```python
from build123d import *

# Parameters (mm, degrees)
ESQUISSE1_W               = 60
ESQUISSE1_H               = 70
T_LE_DE_BASE_PLI_E1_DEPTH = 3
ENL_V_MAT_EXTRU_1_REACH   = 48.195
ESQUISSE6_R               = 2
ENL_V_MAT_EXTRU_2_REACH   = 48.195
ESQUISSE7_R               = 2
BOSS_EXTRU_1_START        = 4
ESQUISSE9_R               = 4
ESQUISSE9_R_2             = 2
BOSS_EXTRU_1_DEPTH        = 4
ENL_V_MAT_EXTRU_3_REACH   = 48.271
ESQUISSE10_W              = 45
ESQUISSE10_H              = 35
BOSS_EXTRU_2_START        = -1
ESQUISSE11_R              = 2
BOSS_EXTRU_2_DEPTH        = 1
BOSS_EXTRU_3_START        = 3
ESQUISSE12_R              = 4
ESQUISSE12_R_2            = 2
BOSS_EXTRU_3_DEPTH        = 3
BOSS_EXTRU_4_START        = 1
ESQUISSE13_R              = 4
BOSS_EXTRU_4_DEPTH        = 1


# Sheet-metal steps are written as plain solids
with BuildPart() as part:
    # Esquisse1 → Tôle de base pliée1 (new body)
    with BuildSketch(Plane.XY):
        Rectangle(ESQUISSE1_W, ESQUISSE1_H)
    extrude(amount=-T_LE_DE_BASE_PLI_E1_DEPTH)

    # Esquisse6 → Enlèv. mat.-Extru.1 (cut, up to next)
    with BuildSketch(Plane.XY, mode=Mode.PRIVATE) as enl_v_mat_extru_1_sk1:
        with Locations((-24.5, 29)):
            Circle(ESQUISSE6_R)
    enl_v_mat_extru_1_tool1 = extrude(enl_v_mat_extru_1_sk1.sketch, amount=-ENL_V_MAT_EXTRU_1_REACH, mode=Mode.PRIVATE) & part.part
    # Esquisse6 → Enlèv. mat.-Extru.1 (cut, up to next)
    with BuildSketch(Plane.XY, mode=Mode.PRIVATE) as enl_v_mat_extru_1_sk2:
        with Locations((24.5, 29)):
            Circle(ESQUISSE6_R)
    enl_v_mat_extru_1_tool2 = extrude(enl_v_mat_extru_1_sk2.sketch, amount=-ENL_V_MAT_EXTRU_1_REACH, mode=Mode.PRIVATE) & part.part
    # Esquisse6 → Enlèv. mat.-Extru.1 (cut, up to next)
    with BuildSketch(Plane.XY, mode=Mode.PRIVATE) as enl_v_mat_extru_1_sk3:
        with Locations((24.5, -29)):
            Circle(ESQUISSE6_R)
    enl_v_mat_extru_1_tool3 = extrude(enl_v_mat_extru_1_sk3.sketch, amount=-ENL_V_MAT_EXTRU_1_REACH, mode=Mode.PRIVATE) & part.part
    # Esquisse6 → Enlèv. mat.-Extru.1 (cut, up to next)
    with BuildSketch(Plane.XY, mode=Mode.PRIVATE) as enl_v_mat_extru_1_sk4:
        with Locations((-24.5, -29)):
            Circle(ESQUISSE6_R)
    enl_v_mat_extru_1_tool4 = extrude(enl_v_mat_extru_1_sk4.sketch, amount=-ENL_V_MAT_EXTRU_1_REACH, mode=Mode.PRIVATE) & part.part
    add(enl_v_mat_extru_1_tool1.solids().sort_by_distance((-24.5, 29, 0))[0], mode=Mode.SUBTRACT)
    add(enl_v_mat_extru_1_tool2.solids().sort_by_distance((24.5, 29, 0))[0], mode=Mode.SUBTRACT)
    add(enl_v_mat_extru_1_tool3.solids().sort_by_distance((24.5, -29, 0))[0], mode=Mode.SUBTRACT)
    add(enl_v_mat_extru_1_tool4.solids().sort_by_distance((-24.5, -29, 0))[0], mode=Mode.SUBTRACT)

    # Esquisse7 → Enlèv. mat.-Extru.2 (cut, up to next)
    with BuildSketch(Plane.XY, mode=Mode.PRIVATE) as enl_v_mat_extru_2_sk1:
        with Locations((-17, -23.75)):
            Circle(ESQUISSE7_R)
    enl_v_mat_extru_2_tool1 = extrude(enl_v_mat_extru_2_sk1.sketch, amount=-ENL_V_MAT_EXTRU_2_REACH, mode=Mode.PRIVATE) & part.part
    # Esquisse7 → Enlèv. mat.-Extru.2 (cut, up to next)
    with BuildSketch(Plane.XY, mode=Mode.PRIVATE) as enl_v_mat_extru_2_sk2:
        with Locations((0, -23.75)):
            Circle(ESQUISSE7_R)
    enl_v_mat_extru_2_tool2 = extrude(enl_v_mat_extru_2_sk2.sketch, amount=-ENL_V_MAT_EXTRU_2_REACH, mode=Mode.PRIVATE) & part.part
    # Esquisse7 → Enlèv. mat.-Extru.2 (cut, up to next)
    with BuildSketch(Plane.XY, mode=Mode.PRIVATE) as enl_v_mat_extru_2_sk3:
        with Locations((17, -23.75)):
            Circle(ESQUISSE7_R)
    enl_v_mat_extru_2_tool3 = extrude(enl_v_mat_extru_2_sk3.sketch, amount=-ENL_V_MAT_EXTRU_2_REACH, mode=Mode.PRIVATE) & part.part
    # Esquisse7 → Enlèv. mat.-Extru.2 (cut, up to next)
    with BuildSketch(Plane.XY, mode=Mode.PRIVATE) as enl_v_mat_extru_2_sk4:
        with Locations((0, 23.75)):
            Circle(ESQUISSE7_R)
    enl_v_mat_extru_2_tool4 = extrude(enl_v_mat_extru_2_sk4.sketch, amount=-ENL_V_MAT_EXTRU_2_REACH, mode=Mode.PRIVATE) & part.part
    # Esquisse7 → Enlèv. mat.-Extru.2 (cut, up to next)
    with BuildSketch(Plane.XY, mode=Mode.PRIVATE) as enl_v_mat_extru_2_sk5:
        with Locations((17, 23.75)):
            Circle(ESQUISSE7_R)
    enl_v_mat_extru_2_tool5 = extrude(enl_v_mat_extru_2_sk5.sketch, amount=-ENL_V_MAT_EXTRU_2_REACH, mode=Mode.PRIVATE) & part.part
    # Esquisse7 → Enlèv. mat.-Extru.2 (cut, up to next)
    with BuildSketch(Plane.XY, mode=Mode.PRIVATE) as enl_v_mat_extru_2_sk6:
        with Locations((-17, 23.75)):
            Circle(ESQUISSE7_R)
    enl_v_mat_extru_2_tool6 = extrude(enl_v_mat_extru_2_sk6.sketch, amount=-ENL_V_MAT_EXTRU_2_REACH, mode=Mode.PRIVATE) & part.part
    add(enl_v_mat_extru_2_tool1.solids().sort_by_distance((-17, -23.75, 0))[0], mode=Mode.SUBTRACT)
    add(enl_v_mat_extru_2_tool2.solids().sort_by_distance((0, -23.75, 0))[0], mode=Mode.SUBTRACT)
    add(enl_v_mat_extru_2_tool3.solids().sort_by_distance((17, -23.75, 0))[0], mode=Mode.SUBTRACT)
    add(enl_v_mat_extru_2_tool4.solids().sort_by_distance((0, 23.75, 0))[0], mode=Mode.SUBTRACT)
    add(enl_v_mat_extru_2_tool5.solids().sort_by_distance((17, 23.75, 0))[0], mode=Mode.SUBTRACT)
    add(enl_v_mat_extru_2_tool6.solids().sort_by_distance((-17, 23.75, 0))[0], mode=Mode.SUBTRACT)

    # Esquisse9 → Boss.-Extru.1 (add)
    # profile 1 of 4: a face of its own
    with BuildSketch(Plane.XY.offset(BOSS_EXTRU_1_START)):
        with Locations((-24.5, 29)):
            Circle(ESQUISSE9_R)
        with Locations((-24.5, 29)):
            Circle(ESQUISSE9_R_2, mode=Mode.SUBTRACT)
    # profile 2 of 4: a face of its own
    with BuildSketch(Plane.XY.offset(BOSS_EXTRU_1_START)):
        with Locations((24.5, 29)):
            Circle(ESQUISSE9_R)
        with Locations((24.5, 29)):
            Circle(ESQUISSE9_R_2, mode=Mode.SUBTRACT)
    # profile 3 of 4: a face of its own
    with BuildSketch(Plane.XY.offset(BOSS_EXTRU_1_START)):
        with Locations((24.5, -29)):
            Circle(ESQUISSE9_R)
        with Locations((24.5, -29)):
            Circle(ESQUISSE9_R_2, mode=Mode.SUBTRACT)
    # profile 4 of 4: a face of its own
    with BuildSketch(Plane.XY.offset(BOSS_EXTRU_1_START)):
        with Locations((-24.5, -29)):
            Circle(ESQUISSE9_R)
        with Locations((-24.5, -29)):
            Circle(ESQUISSE9_R_2, mode=Mode.SUBTRACT)
    extrude(amount=-BOSS_EXTRU_1_DEPTH)

    # Esquisse10 → Enlèv. mat.-Extru.3 (cut, up to next)
    with BuildSketch(Plane.XY, mode=Mode.PRIVATE) as enl_v_mat_extru_3_sk1:
        Rectangle(ESQUISSE10_W, ESQUISSE10_H)
    enl_v_mat_extru_3_tool1 = extrude(enl_v_mat_extru_3_sk1.sketch, amount=-ENL_V_MAT_EXTRU_3_REACH, mode=Mode.PRIVATE) & part.part
    add(enl_v_mat_extru_3_tool1.solids().sort_by_distance((0, 0, 0))[0], mode=Mode.SUBTRACT)

    # Esquisse11 → Boss.-Extru.2 (add)
    with BuildSketch(Plane(origin=(0, 0, -3), x_dir=(-1, 0, 0), z_dir=(0, 0, -1)).offset(BOSS_EXTRU_2_START)):
        with Locations(Location((-24.5, -29, 0), (0, 0, 180))):
            Circle(ESQUISSE11_R)
        with Locations(Location((24.5, -29, 0), (0, 0, 180))):
            Circle(ESQUISSE11_R)
        with Locations(Location((24.5, 29, 0), (0, 0, 180))):
            Circle(ESQUISSE11_R)
        with Locations(Location((-24.5, 29, 0), (0, 0, 180))):
            Circle(ESQUISSE11_R)
    extrude(amount=BOSS_EXTRU_2_DEPTH)

    # Esquisse12 → Boss.-Extru.3 (add)
    # profile 1 of 6: a face of its own
    with BuildSketch(Plane.XY.offset(BOSS_EXTRU_3_START)):
        with Locations((-17, 23.75)):
            Circle(ESQUISSE12_R)
        with Locations((-17, 23.75)):
            Circle(ESQUISSE12_R_2, mode=Mode.SUBTRACT)
    # profile 2 of 6: a face of its own
    with BuildSketch(Plane.XY.offset(BOSS_EXTRU_3_START)):
        with Locations((0, 23.75)):
            Circle(ESQUISSE12_R)
        with Locations((0, 23.75)):
            Circle(ESQUISSE12_R_2, mode=Mode.SUBTRACT)
    # profile 3 of 6: a face of its own
    with BuildSketch(Plane.XY.offset(BOSS_EXTRU_3_START)):
        with Locations((17, 23.75)):
            Circle(ESQUISSE12_R)
        with Locations((17, 23.75)):
            Circle(ESQUISSE12_R_2, mode=Mode.SUBTRACT)
    # profile 4 of 6: a face of its own
    with BuildSketch(Plane.XY.offset(BOSS_EXTRU_3_START)):
        with Locations((17, -23.75)):
            Circle(ESQUISSE12_R)
        with Locations((17, -23.75)):
            Circle(ESQUISSE12_R_2, mode=Mode.SUBTRACT)
    # profile 5 of 6: a face of its own
    with BuildSketch(Plane.XY.offset(BOSS_EXTRU_3_START)):
        with Locations((0, -23.75)):
            Circle(ESQUISSE12_R)
        with Locations((0, -23.75)):
            Circle(ESQUISSE12_R_2, mode=Mode.SUBTRACT)
    # profile 6 of 6: a face of its own
    with BuildSketch(Plane.XY.offset(BOSS_EXTRU_3_START)):
        with Locations((-17, -23.75)):
            Circle(ESQUISSE12_R)
        with Locations((-17, -23.75)):
            Circle(ESQUISSE12_R_2, mode=Mode.SUBTRACT)
    extrude(amount=-BOSS_EXTRU_3_DEPTH)

    # Esquisse13 → Boss.-Extru.4 (add)
    with BuildSketch(Plane.XY.offset(3).offset(BOSS_EXTRU_4_START)):
        with Locations((-17, -23.75)):
            Circle(ESQUISSE13_R)
        with Locations((0, -23.75)):
            Circle(ESQUISSE13_R)
        with Locations((17, -23.75)):
            Circle(ESQUISSE13_R)
        with Locations((17, 23.75)):
            Circle(ESQUISSE13_R)
        with Locations((0, 23.75)):
            Circle(ESQUISSE13_R)
        with Locations((-17, 23.75)):
            Circle(ESQUISSE13_R)
    extrude(amount=-BOSS_EXTRU_4_DEPTH)


solid = part.part
```
Design review of the part built by this model. Coordinates are the model's own, in mm. A direction names the side the tool comes from. Round coordinates to 2 decimals unless told otherwise and drop trailing zeros. Write each loop counter-clockwise with the first axis right and the second up, starting at its lowest first coordinate (ties: lowest second). Pieces come first, ordered by that corner, then holes. Notation, with made-up numbers: (5, 17.5) -> (56, 17.5) arc R18 cw to (56, 49.5) -> close; hole circle Ø1 at (-0.5, 87). An arc over 180 degrees is marked (long way). Write item = value, one per line. Start each with the question number.
1) Take a section at C-C, the plane y = 0.5. State the section outline as (x, z) points, plus the area to 3 significant figures.
2) Mouldability with a two-part tool opening along X and no side actions: class faces 4 (the face through (-25.021, 32.966, 2.028)), 5 (the face through (-30, 0, -1)), 6 (the face through (-17, 24, 3)), 7 (the face through (17, 24, 4)) as +X half, -X half, draft (parallel to the pull), parting line (faces both ways), or undercut.
3) Take a section at B-B, the plane x = 0. State the section outline as (y, z) points, plus the area to 3 significant figures.
4) Tool access review of faces 1 (the face through (22.5, 0, -1)), 2 (the face through (0, -24, 3)), 3 (the face through (-24.934, -30.952, 1.042)): name each direction out of +Z, -Z, +X, -X, +Y, -Y from which nothing blocks a thin tool from reaching the whole face with its end or side.
5) Take a section at A-A, the plane z = 0.75. Count the separate pieces of the cut face and the enclosed holes in it, plus the area to 3 significant figures.
6) Clearance check with flat-ended pins moving along their axes: pin 1 (1 mm diameter, centred on x = -23, y = 0, fed in from +Z); pin 2 (2.5 mm diameter, centred on x = -17, y = 23.75, fed in from -Z); pin 3 (1 mm diameter, centred on x = -19.5, z = 1.5, fed in from -Y). State where each tip first meets the part, or that it passes through.
7) Take a section at D-D, the plane x = -24.5. State the section outline as (y, z) points.
8) Wall thickness on probe 1 along Y at (x, z) = (0, 0.45); probe 2 along Y at (x, z) = (-24.5, 1.25); probe 3 along Y at (x, z) = (24.5, -0.4): over which ranges is each line inside the solid? List them lowest first. Write a range as from..to.
Results list:
q1.outline = (-30, -3) -> (-22.5, -3) -> (-22.5, 0) -> (-30, 0) -> close; (22.5, -3) -> (30, -3) -> (30, 0) -> (22.5, 0) -> close
q1.area = 45.0 mm²
q2.face_4 = undercut
q2.face_5 = -X half
q2.face_6 = undercut
q2.face_7 = draft
q3.outline = (-35, -3) -> (-25.75, -3) -> (-25.75, 3) -> (-21.75, 3) -> (-21.75, -3) -> (-17.5, -3) -> (-17.5, 0) -> (-19.75, 0) -> (-19.75, 4) -> (-27.75, 4) -> (-27.75, 0) -> (-35, 0) -> close; (17.5, -3) -> (21.75, -3) -> (21.75, 3) -> (25.75, 3) -> (25.75, -3) -> (35, -3) -> (35, 0) -> (27.75, 0) -> (27.75, 4) -> (19.75, 4) -> (19.75, 0) -> (17.5, 0) -> close
q3.area = 121 mm²
q4.face_1 = +Z, -Z
q4.face_2 = -Z
q4.face_3 = +Z
q5.separate_pieces = 10
q5.enclosed_holes = 10
q5.area = 377 mm²
q6.pin_1 = 0
q6.pin_2 = 3
q6.pin_3 = -27.21
q7.outline = (-35, -3) -> (35, -3) -> (35, 0) -> (33, 0) -> (33, 4) -> (31, 4) -> (31, -2) -> (27, -2) -> (27, 4) -> (25, 4) -> (25, 0) -> (-25, 0) -> (-25, 4) -> (-27, 4) -> (-27, -2) -> (-31, -2) -> (-31, 4) -> (-33, 4) -> (-33, 0) -> (-35, 0) -> close
q8.probe_1 = -27.75..-25.75, -21.75..-19.75, 19.75..21.75, 25.75..27.75
q8.probe_2 = -33..-31, -27..-25, 25..27, 31..33
q8.probe_3 = -35..-31, -27..27, 31..35
